The listing builds one solid part. Answer for the finished solid, in the listing's coordinates (mm). Face numbers are marked on the shaded views. Round coordinates to 2 decimals unless told otherwise and drop trailing zeros. Order: outer loops, then holes, each group sorted by start corner. A loop starts at its lowest first (then second) coordinate and runs counter-clockwise, first axis right, second up. Notation, with made-up numbers: M 33.5,85 L 83.5,85 A21 cw 83.5,117 Z; hole C -6.5,-23.75 d6. An arc over 180 degrees is marked long. Put each result on its own line as item: value. Start each with the question number.
1. The part is cut by section B-B (y = 65). Give the vertices of the cut face in (x, z), then the cut area to 3 significant figures.
2. Each of these flat-tipped pins is pushed along its axis until it touches: pin 1 Ø1 at (x, z) = (144, 1.5) entering from +Y; pin 2 Ø10 at (x, y) = (37, 41) entering from -Z; pin 3 Ø1 at (x, z) = (35.5, 3) entering from +Y; pin 4 Ø1.5 at (x, z) = (71, 3.5) entering from +Y. Where does it stop, or does it pass through?
3. The part is cut by section A-A (z = 1.3). Give the vertices of the cut face in (x, y).
4. The mould has two halves that part along Z. Classify the marked faces 1 and 2: +Z half, -Z half, draft (parallel to the pull), parting line (faces both ways), or undercut.
5. Consider line 1 (X direction, y = 4, z = 3.45); line 2 (Y direction, x = 29, z = 3.1); line 3 (Y direction, x = 170.5, z = 4.6) (3 decimals). Determine where each line is inside the solid, lowest interval first.
6. The part is cut by section C-C (x = 86.5). Give the vertices of the cut face in (y, z), then the cut area to 3 significant figures.
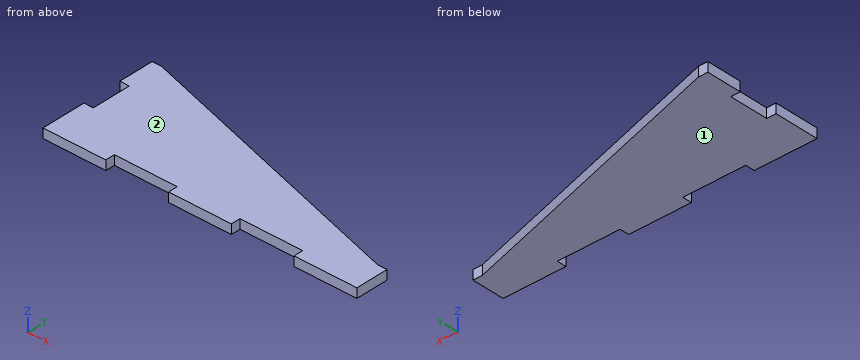
Autodesk Inventor part; units mm, degrees
ref_plane "YZ Plane" through (0, 0, 0) normal (1, 0, 0) x (0, 1, 0)
ref_plane "XZ Plane" through (0, 0, 0) normal (0, 1, 0) x (-1, 0, 0)
ref_plane "XY Plane" through (0, 0, 0) normal (0, 0, 1) x (1, 0, 0)
ref_plane "Work Plane1" through (0, 0, 0) normal (0, 0, 1) x (1, 0, 0)
sketch "Sketch1" plane through (0, 0, 0) normal (0, 0, 1) x (1, 0, 0)
  line L0 (0, 6) -> (40, 6)
  line L1 (0, 0) -> (0, 6)
  line L2 (40, 0) -> (0, 0)
  line L3 (40, 0) -> (40, 6)
  line L4 (80, 0) -> (80, 6)
  line L5 (80, 6) -> (40, 6)
  line L6 (40, 6) -> (40, 0)
  line L7 (40, 0) -> (80, 0)
  line L8 (80, 6) -> (120, 6)
  line L9 (80, 0) -> (80, 6)
  line L10 (120, 0) -> (80, 0)
  line L11 (120, 0) -> (120, 6)
  line L12 (160, 0) -> (160, 6)
  line L13 (160, 6) -> (120, 6)
  line L14 (120, 6) -> (120, 0)
  line L15 (120, 0) -> (160, 0)
  line L16 (160, 6) -> (200, 6)
  line L17 (160, 0) -> (160, 6)
  line L18 (200, 0) -> (160, 0)
  line L19 (200, 6) -> (200, 0)
  line L20 (200, 6) -> (200, 21)
  line L21 (194, 21) -> (200, 21)
  line L22 (194, 21) -> (194, 6)
  line L23 (194, 6) -> (200, 6)
  line L24 (6, 28.5) -> (0, 28.5)
  line L25 (0, 28.5) -> (0, 6)
  line L26 (6, 6) -> (0, 6)
  line L27 (6, 6) -> (6, 28.5)
  line L28 (0, 53.5) -> (0, 28.5)
  line L29 (6, 28.5) -> (0, 28.5)
  line L30 (6, 28.5) -> (6, 53.5)
  line L31 (6, 53.5) -> (0, 53.5)
  line L32 (6, 53.5) -> (0, 53.5)
  line L33 (6, 53.5) -> (6, 76)
  line L34 (6, 76) -> (0, 76)
  line L35 (0, 76) -> (0, 53.5)
  line L36 (6, 76) -> (194, 21)
extrude "Plate1" add sketch "Sketch1" along normal blind 6 contours L25 L24 L27 L0 | L0 L3 L2 L1 | L27 L30 L33 L36 L22 L16 L13 L8 L5 L0 | L35 L34 L33 L31 | L8 L11 L10 L4 | L16 L19 L18 L12 | L21 L20 L16 L22
equation "\"d0\" = Thickness"
equation "\"BendRadius\" = Thickness"
equation "\"BendReliefWidth\" = Thickness"
equation "\"BendReliefDepth\" = 0.5 * Thickness"
equation "\"CornerReliefSize\" = 4 * Thickness"
equation "\"MinimumRemnant\" = 2 * Thickness"
equation "\"TransitionRadius\" = BendRadius"
equation "\"JacobiRadiusSize\" = BendRadius"
equation "\"GapSize\" = Thickness"
properties material "Wood (Birch)"
Resolved:
1. outline: M 0,0 L 43.6,0 L 43.6,6 L 0,6 Z
1. area: 262 mm2
2. pin 1: y = 35.77
2. pin 2: z = 0
2. pin 3: y = 67.52
2. pin 4: y = 57.2
3. outline: M 0,0 L 40,0 L 40,6 L 80,6 L 80,0 L 120,0 L 120,6 L 160,6 L 160,0 L 200,0 L 200,21 L 194,21 L 6,76 L 0,76 L 0,53.5 L 6,53.5 L 6,28.5 L 0,28.5 Z
4. face 1: -Z half
4. face 2: +Z half
5. line 1: 0 to 40, 80 to 120, 160 to 200
5. line 2: 0 to 69.27
5. line 3: 0 to 27.875
6. outline: M 0,0 L 52.45,0 L 52.45,6 L 0,6 Z
6. area: 315 mm2
